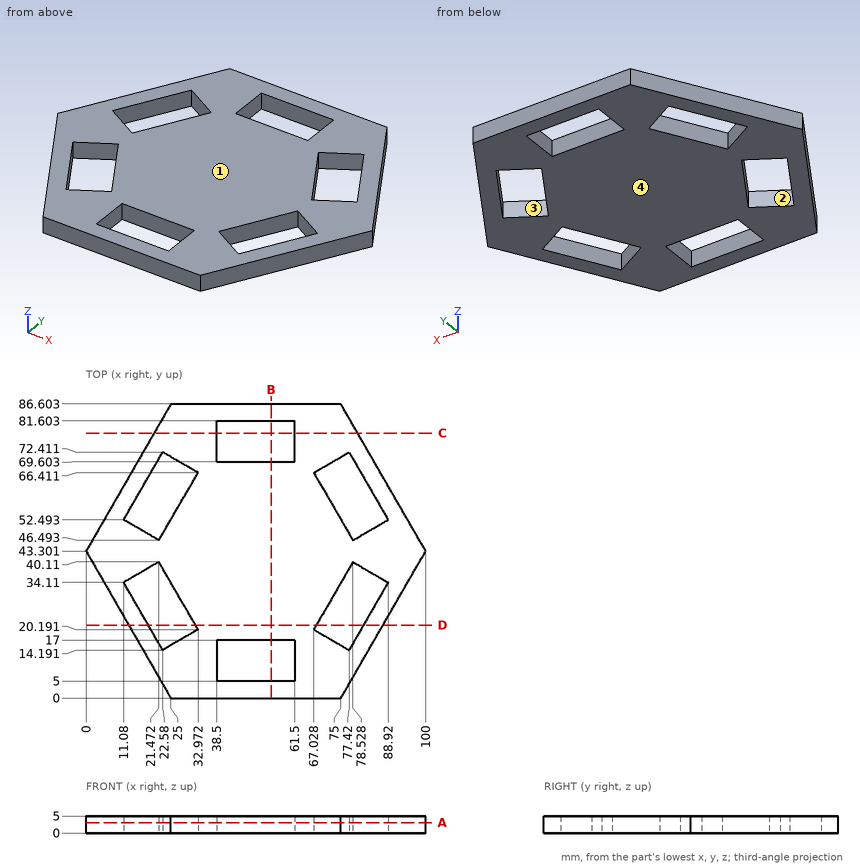
Verification items for this drawing (mm, ordinates from the low corner). A direction names the side the tool comes from. Coordinates: 2 decimals unless noted, no trailing zeros. Loops run counter-clockwise (first coordinate to the right, second up) from the corner with the lowest first, then second, coordinate; pieces in that order, holes last.
Item 1: Go/stop test with flat-tipped pins: pin 1 Ø2.5 at (y, z) = (8, 3.5) entering from +X; pin 2 Ø1.5 at (y, z) = (41.5, 3.5) entering from -X; pin 3 Ø2.5 at (y, z) = (76, 2) entering from -X. Record where each tip stops, or that it passes through.
Item 2: Sectioned sample at D-D, the plane y = 21.5. Record the boundary of the cut face in (x, z).
Item 3: Thickness scan on line 1 (Y direction, x = 44.5, z = 0.95); line 2 (Y direction, x = 80, z = 1.05) (1 decimal); line 3 (X direction, y = 52.5, z = 3.35) (1 decimal). Record the ranges inside material, lowest first.
Item 4: Access from +Z, -Z, +X, -X, +Y, -Y to the whole of each face (thin tool, end or side, straight path). Record for the marked faces 1 and 2.
Item 5: Release check for a two-part mould opening along X. For the marked faces 3 and 4 record: released by +X, released by -X, zero draft, split by the parting line, or undercut.
Item 6: Sectioned sample at A-A, the plane z = 3.15. Count the separate pieces of the cut face and the enclosed holes in it, then the cut area to 3 significant figures.
Item 7: Sectioned sample at C-C, the plane y = 78. Record the boundary of the cut face in (x, z), then the cut area to 3 significant figures.
Item 8: Sectioned sample at B-B, the plane x = 54.5. Record the boundary of the cut face in (y, z).
Check result:
1. pin 1: stops at x = 80.34
1. pin 2: stops at x = 0.61
1. pin 3: stops at x = 18.16
2. outline: (12.59, 0) - (18.36, 0) - (18.36, 5) - (12.59, 5) - close; (32.22, 0) - (67.78, 0) - (67.78, 5) - (32.22, 5) - close; (81.64, 0) - (87.41, 0) - (87.41, 5) - (81.64, 5) - close
3. line 1: y = 0 to 5, 17 to 69.6, 81.6 to 86.6
3. line 2: y = 8.7 to 18.7, 39.3 to 47.3, 67.9 to 77.9
3. line 3: x = 5.3 to 11.1, 24.9 to 75.1, 88.9 to 94.7
4. face 1: +Z, +X, -X, +Y, -Y
4. face 2: +Z, -Z
5. face 3: undercut
5. face 4: zero draft
6. separate pieces: 1
6. enclosed holes: 6
6. area: 4,840 mm2
7. outline: (20.03, 0) - (38.5, 0) - (38.5, 5) - (20.03, 5) - close; (61.5, 0) - (79.97, 0) - (79.97, 5) - (61.5, 5) - close
7. area: 185 mm2
8. outline: (0, 0) - (5, 0) - (5, 5) - (0, 5) - close; (17, 0) - (69.6, 0) - (69.6, 5) - (17, 5) - close; (81.6, 0) - (86.6, 0) - (86.6, 5) - (81.6, 5) - close
